```python
from build123d import *

# Parameters (mm, degrees)
SKETCH_1_R          = 25
SKETCH_1_R_2        = 1.6
SKETCH_1_R_3        = 2.1
EXTRUDE_1_DEPTH     = 2.5
SKETCH_3_R          = 2.5
CUT_EXTRUDE_1_DEPTH = 10
SKETCH_4_R          = 2.1
CUT_EXTRUDE_2_DEPTH = 10
SKETCH_5_W          = 20
SKETCH_5_H          = 5
EXTRUDE_2_DEPTH     = 5
CUT_EXTRUDE_3_DEPTH = 97.176920308
FILLET_1_R          = 5


with BuildPart() as part:
    # 草图1 → 凸台-拉伸1 (new, symmetric)
    with BuildSketch(Plane(origin=(0, 0, 0), x_dir=(1, 0, 0), z_dir=(0, 1, 0))):
        with BuildLine():
            Line((-60, 0), (-60, -70))
            Line((-60, -70), (60, -70))
            Line((60, -70), (60, 0))
            ThreePointArc((60, 0), (42.426406871, 42.426406871), (0, 60))
            ThreePointArc((0, 60), (-42.426406871, 42.426406871), (-60, 0))
        make_face()
        with Locations(Location((0, 0, 0), (0, 0, 270))):
            Circle(SKETCH_1_R, mode=Mode.SUBTRACT)
        with Locations(Location((-40, -57.62, 0), (0, 0, 270))):
            Circle(SKETCH_1_R_2, mode=Mode.SUBTRACT)
        with Locations(Location((40, -57.62, 0), (0, 0, 90))):
            Circle(SKETCH_1_R_2, mode=Mode.SUBTRACT)
        with Locations(Location((-37.5, 0, 0), (0, 0, 270))):
            Circle(SKETCH_1_R_2, mode=Mode.SUBTRACT)
        with Locations(Location((-28.726666617, 24.104535363, 0), (0, 0, 270))):
            Circle(SKETCH_1_R_2, mode=Mode.SUBTRACT)
        with Locations(Location((-6.511806663, 36.930290738, 0), (0, 0, 270))):
            Circle(SKETCH_1_R_2, mode=Mode.SUBTRACT)
        with Locations(Location((18.75, 32.475952642, 0), (0, 0, 270))):
            Circle(SKETCH_1_R_2, mode=Mode.SUBTRACT)
        with Locations(Location((35.238473279, 12.825755375, 0), (0, 0, 270))):
            Circle(SKETCH_1_R_2, mode=Mode.SUBTRACT)
        with Locations(Location((35.238473279, -12.825755375, 0), (0, 0, 270))):
            Circle(SKETCH_1_R_2, mode=Mode.SUBTRACT)
        with Locations(Location((18.75, -32.475952642, 0), (0, 0, 270))):
            Circle(SKETCH_1_R_2, mode=Mode.SUBTRACT)
        with Locations(Location((-6.511806663, -36.930290738, 0), (0, 0, 270))):
            Circle(SKETCH_1_R_2, mode=Mode.SUBTRACT)
        with Locations(Location((-28.726666617, -24.104535363, 0), (0, 0, 270))):
            Circle(SKETCH_1_R_2, mode=Mode.SUBTRACT)
        with Locations(Location((-11, -65, 0), (0, 0, 270))):
            Circle(SKETCH_1_R_3, mode=Mode.SUBTRACT)
        with Locations(Location((11, -65, 0), (0, 0, 90))):
            Circle(SKETCH_1_R_3, mode=Mode.SUBTRACT)
        with Locations(Location((0, -54, 0), (0, 0, 270))):
            Circle(SKETCH_1_R_2, mode=Mode.SUBTRACT)
        with Locations(Location((8.488193337, 40, 0), (0, 0, 270))):
            Circle(SKETCH_1_R_2, mode=Mode.SUBTRACT)
        with Locations(Location((-1.511806663, 40.862744239, 0), (0, 0, 270))):
            Circle(SKETCH_1_R_2, mode=Mode.SUBTRACT)
        with Locations(Location((-11.420717282, 39.263426275, 0), (0, 0, 270))):
            Circle(SKETCH_1_R_2, mode=Mode.SUBTRACT)
    extrude(amount=EXTRUDE_1_DEPTH, both=True)

    # 草图3 → 切除-拉伸1 (cut)
    with BuildSketch(Plane(origin=(0, 2.5, 0), x_dir=(1, 0, 0), z_dir=(0, 1, 0))):
        with Locations(Location((-27.251086003, -9.918584156, 0), (0, 0, 270))):
            Circle(SKETCH_3_R)
        with Locations(Location((-14.5, 25.11473671, 0), (0, 0, 270))):
            Circle(SKETCH_3_R)
        with Locations(Location((5.035797152, 28.559424837, 0), (0, 0, 270))):
            Circle(SKETCH_3_R)
        with Locations(Location((22.21528885, 18.640840681, 0), (0, 0, 270))):
            Circle(SKETCH_3_R)
        with Locations(Location((29, 0, 0), (0, 0, 270))):
            Circle(SKETCH_3_R)
        with Locations(Location((22.21528885, -18.640840681, 0), (0, 0, 270))):
            Circle(SKETCH_3_R)
        with Locations(Location((5.035797152, -28.559424837, 0), (0, 0, 270))):
            Circle(SKETCH_3_R)
        with Locations(Location((-14.5, -25.11473671, 0), (0, 0, 270))):
            Circle(SKETCH_3_R)
        with Locations(Location((-27.251086003, 9.918584156, 0), (0, 0, 270))):
            Circle(SKETCH_3_R)
    extrude(amount=-CUT_EXTRUDE_1_DEPTH, mode=Mode.SUBTRACT)

    # 草图4 → 切除-拉伸2 (cut)
    with BuildSketch(Plane(origin=(0, 2.5, 0), x_dir=(1, 0, 0), z_dir=(0, 1, 0))):
        with Locations(Location((-40, -47.62, 0), (0, 0, 270))):
            Circle(SKETCH_4_R)
        with Locations(Location((-40, -37.62, 0), (0, 0, 270))):
            Circle(SKETCH_4_R)
        with Locations(Location((-40, -27.62, 0), (0, 0, 270))):
            Circle(SKETCH_4_R)
        with Locations(Location((40, -47.62, 0), (0, 0, 270))):
            Circle(SKETCH_4_R)
        with Locations(Location((40, -37.62, 0), (0, 0, 270))):
            Circle(SKETCH_4_R)
        with Locations(Location((40, -27.62, 0), (0, 0, 270))):
            Circle(SKETCH_4_R)
    extrude(amount=-CUT_EXTRUDE_2_DEPTH, mode=Mode.SUBTRACT)

    # 草图5 → 凸台-拉伸2 (add)
    with BuildSketch(Plane.XY.offset(70)):
        with Locations((40, 0)):
            Rectangle(SKETCH_5_W, SKETCH_5_H)
        with Locations((-40, 0)):
            Rectangle(SKETCH_5_W, SKETCH_5_H)
    extrude(amount=EXTRUDE_2_DEPTH)

    # 草图7 → 切除-拉伸3 (cut, through all)
    with BuildSketch(Plane(origin=(0, 2.5, 0), x_dir=(1, 0, 0), z_dir=(0, 1, 0))):
        with BuildLine():
            Line((-41.406951107, -17.62), (-60, -70))
            Line((-60, -70), (-60, 0))
            ThreePointArc((-60, 0), (0, 60), (60, 0))
            Line((60, 0), (60, -70))
            Line((60, -70), (41.406951107, -17.62))
            ThreePointArc((41.406951107, -17.62), (0, 45), (-41.406951107, -17.62))
        make_face()
    extrude(amount=-CUT_EXTRUDE_3_DEPTH, mode=Mode.SUBTRACT)

    # 圆角1
    fillet_1_edges = [part.edges().sort_by_distance(p)[0] for p in [
        (60, 0, 70),
        (-60, 0, 70),
    ]]
    fillet(fillet_1_edges, radius=FILLET_1_R)


solid = part.part
```
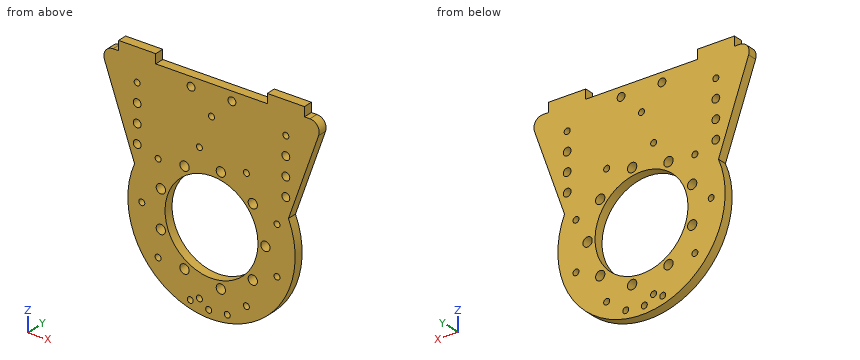
The listing builds one solid part. Answer for the finished solid, in the listing's coordinates (mm). Give positions to 0.01 mm unless a question says otherwise; leave off trailing zeros. Loops run counter-clockwise (first coordinate to the right, second up) from the corner with the lowest first, then second, coordinate; pieces in that order, holes last. Notation, with made-up numbers: M -6,19.25 L 10,19.25 A31 ccw 10,52.25 Z; hole C 62,1 d3. An arc over 180 degrees is marked long. One line per item, written item: value.
1. Section C-C on y = 1.4 is taken. State how many separate pieces and enclosed holes the cut face has, plus the area to 3 significant figures.
Found:
separate pieces: 1
enclosed holes: 33
area: 7,840 mm^2
2. This flat-tipped pin is pushed along its axis until it touches: P1, Ø5.5, axis at x = 40, z = 47.62, coming from the -Y side. Where does it stop, or does it pass through?
Found:
P1: y = -2.5
3. Section A-A on z = 65 is taken. Determine the outline of the cut face in (x, y), plus the area to 3 significant figures.
Found:
outline: M -57.92,-2.5 L -13.1,-2.5 L -13.1,2.5 L -57.92,2.5 Z; M -8.9,-2.5 L 8.9,-2.5 L 8.9,2.5 L -8.9,2.5 Z; M 13.1,-2.5 L 57.92,-2.5 L 57.92,2.5 L 13.1,2.5 Z
area: 537 mm^2
4. Find the intervals of material crossed by probe 1 along X at (y, z) = (0.7, 0); probe 2 along X at (y, z) = (-1.9, 9); probe 3 along X at (y, z) = (-0.15, 57.62), in increasing order.
Found:
probe 1: -45 to -39.1, -35.9 to -25, 25 to 26.5, 31.5 to 45
probe 2: -44.09 to -29.58, -24.93 to -23.32, 23.32 to 44.09
probe 3: -55.61 to -41.6, -38.4 to 38.4, 41.6 to 55.61
5. Section D-D on x = -34 is taken. Determine the outline of the cut face in (y, z), plus the area to 3 significant figures.
Found:
outline: M -2.5,-29.48 L 2.5,-29.48 L 2.5,75 L -2.5,75 Z
area: 522 mm^2
6. Section B-B on z = 47.62 is taken. Determine the outline of the cut face in (x, y), plus the area to 3 significant figures.
Found:
outline: M -52.06,-2.5 L -42.1,-2.5 L -42.1,2.5 L -52.06,2.5 Z; M -37.9,-2.5 L 37.9,-2.5 L 37.9,2.5 L -37.9,2.5 Z; M 42.1,-2.5 L 52.06,-2.5 L 52.06,2.5 L 42.1,2.5 Z
area: 479 mm^2
